Work out the finished part from the listing and answer in its coordinate system (mm). Round coordinates to 2 decimals unless told otherwise and drop trailing zeros. Write each loop counter-clockwise with the first axis right and the second up, starting at its lowest first coordinate (ties: lowest second). Pieces come first, ordered by that corner, then holes. Notation, with made-up numbers: M -6,-26.5 L 15,-26.5 A23 ccw 15,-8.5 Z; hole C 49,0 d1. An arc over 180 degrees is marked long. Answer in a Markdown table with one row per item.
```python
from build123d import *

# Parameters (mm, degrees)
BOSS_EXTRUDE1_DEPTH = 3.175
SKETCH3_W           = 3.175
SKETCH3_H           = 16.163636364
CUT_EXTRUDE2_DEPTH  = 10
SKETCH4_W           = 16.16
SKETCH4_H           = 3.175
CUT_EXTRUDE3_DEPTH  = 10


with BuildPart() as part:
    # Sketch1 → Boss-Extrude1 (new body)
    with BuildSketch(Plane.XY):
        Polygon((0, 50.8), (-3.175, 50.8), (-3.175, 0), (58.175, 0), (58.175, 50.8), (55, 50.8), (55, 66.963636364), (58.175, 66.963636364), (58.175, 83.12), (55, 83.12), (55, 99.283636364), (58.175, 99.283636364), (58.175, 115.44), (55, 115.44), (55, 131.603636364), (58.175, 131.603636364), (58.175, 147.76), (55, 147.76), (55, 163.923636364), (58.175, 163.923636364), (58.175, 180.08), (55, 180.08), (55, 196.243636364), (58.175, 196.243636364), (58.175, 212.4), (55, 212.4), (55, 228.563636364), (58.175, 228.563636364), (58.175, 244.72), (55, 244.72), (55, 260.883636364), (58.175, 260.883636364), (58.175, 279.4), (-3.175, 279.4), (-3.175, 260.883636364), (0, 260.883636364), (0, 244.72), (-3.175, 244.72), (-3.175, 228.563636364), (0, 228.563636364), (0, 212.4), (-3.175, 212.4), (-3.175, 196.243636364), (0, 196.243636364), (0, 180.109090909), (0, 180.08), (-3.175, 180.08), (-3.175, 163.923636364), (0, 163.923636364), (0, 147.76), (-3.175, 147.76), (-3.175, 131.603636364), (0, 131.603636364), (0, 115.44), (-3.175, 115.44), (-3.175, 99.283636364), (0, 99.283636364), (0, 83.12), (-3.175, 83.12), (-3.175, 66.963636364), (0, 66.963636364), align=None)
    extrude(amount=BOSS_EXTRUDE1_DEPTH)

    # Sketch3 → Cut-Extrude2 (cut)
    with BuildSketch(Plane.XY.offset(3.175)):
        with Locations((5.5875, 58.881818182)):
            Rectangle(SKETCH3_W, SKETCH3_H)
        with Locations((5.5875, 91.201818182)):
            Rectangle(SKETCH3_W, SKETCH3_H)
        with Locations((5.5875, 123.521818182)):
            Rectangle(SKETCH3_W, SKETCH3_H)
        with Locations((5.5875, 155.841818182)):
            Rectangle(SKETCH3_W, SKETCH3_H)
        with Locations((5.5875, 188.161818182)):
            Rectangle(SKETCH3_W, SKETCH3_H)
        with Locations((5.5875, 220.481818182)):
            Rectangle(SKETCH3_W, SKETCH3_H)
        with Locations((5.5875, 252.801818182)):
            Rectangle(SKETCH3_W, SKETCH3_H)
    extrude(amount=-CUT_EXTRUDE2_DEPTH, mode=Mode.SUBTRACT)

    # Sketch4 → Cut-Extrude3 (cut)
    with BuildSketch(Plane.XY.offset(3.175)):
        with Locations((31.0875, 106.5875)):
            Rectangle(SKETCH4_W, SKETCH4_H)
    extrude(amount=-CUT_EXTRUDE3_DEPTH, mode=Mode.SUBTRACT)


solid = part.part
```
1. Consider line 1 along X through (y, z) = (95, 1.55) (3 decimals); line 2 along Y through (x, z) = (29.5, 1.5) (3 decimals). Determine where each line is inside the solid, lowest interval first. Write a range as from..to.
Calculated:
| item | result |
|---|---|
| line 1 | x = 0..4, 7.175..55 |
| line 2 | y = 0..105, 108.175..279.4 |
2. The part is cut by section B-B (z = 0.95). Count the separate pieces of the cut face and the enclosed holes in it, plus the area to 3 significant figures.
Calculated:
| item | result |
|---|---|
| separate pieces | 1 |
| enclosed holes | 8 |
| area | 16,000 mm² |
3. Determine the mould class of faces 1 (the flat face through (27, 142, 3.175)), 2 (the flat face through (27, 142, 0)) for opening direction Z: released by +Z, released by -Z, zero draft, split by the parting line, or undercut.
Calculated:
| item | result |
|---|---|
| face 1 | released by +Z |
| face 2 | released by -Z |
4. The part is cut by section A-A (y = 252). Determine the outline of the cut face in (x, z) (3 decimals), plus the area to 3 significant figures.
Calculated:
| item | result |
|---|---|
| outline | M 0,0 L 4,0 L 4,3.175 L 0,3.175 Z; M 7.175,0 L 55,0 L 55,3.175 L 7.175,3.175 Z |
| area | 165 mm² |
5. Given pin 1 (1.6 mm diameter, centred on y = 155.5, z = 1, fed in from +X), flat-ended and moving along its own axis, determine where the tip first touches the part or whether it passes through.
Calculated:
| item | result |
|---|---|
| pin 1 | stops at x = 55 |
